from build123d import *

# Parameters (mm, degrees)
SKETCH001_R  = 35
PAD_DEPTH    = 10
FILLET_R     = 3
SKETCH_R     = 33.5
POCKET_DEPTH = 9
FILLET001_R  = 2


with BuildPart() as part:
    # Sketch001 → Pad (new body)
    with BuildSketch(Plane.XY):
        Circle(SKETCH001_R)
    extrude(amount=PAD_DEPTH)

    # Fillet
    fillet_edges = [part.edges().sort_by_distance(p)[0] for p in [
        (-35, 0, 10),
    ]]
    fillet(fillet_edges, radius=FILLET_R)

    # Sketch → Pocket (cut)
    with BuildSketch(Plane.XY):
        Circle(SKETCH_R)
    extrude(amount=POCKET_DEPTH, mode=Mode.SUBTRACT)

    # Fillet001
    fillet001_edges = [part.edges().sort_by_distance(p)[0] for p in [
        (-33.5, 0, 9),
    ]]
    fillet(fillet001_edges, radius=FILLET001_R)


solid = part.part
Geometry check sheet. Reference: the model listing, model coordinates, mm. A direction names the side the tool comes from. Coordinates: 2 decimals unless noted, no trailing zeros. Loops run counter-clockwise (first coordinate to the right, second up) from the corner with the lowest first, then second, coordinate; pieces in that order, holes last. Notation, with made-up numbers: (22.5, 52) - (41.5, 52) arc R19 cw to (41.5, 80) - close; hole circle Ø3 at (78.25, 8). An arc over 180 degrees is marked (long way). Use one line per item in the form item = value. Start each with the question number.
Item 1: Section check A-A, the plane x = 0. Enter the section's corners in (y, z).
Item 2: Gauge pin test, flat ends, axial feed: pin 1 (19 mm diameter, centred on x = 2, y = 3.5, fed in from -Z); pin 2 (1.5 mm diameter, centred on x = 20, z = 5.5, fed in from +Y); pin 3 (1.5 mm diameter, centred on y = 5, z = 2.5, fed in from -X). Record the tip position at first contact, or that the pin passes through.
Item 3: Thickness scan on probe 1 along Y at (x, z) = (0, 2.25); probe 2 along Z at (x, y) = (-5.5, 12); probe 3 along X at (y, z) = (-19, 1). Record the ranges inside material, lowest first.
Item 4: Tool access check on faces 1 (the face through (0, 0, 10)), 2 (the face through (-7.262, -32.703, 3.451)). Record the directions out of +Z, -Z, +X, -X, +Y, -Y that give a thin tool (end or side, any length) a straight path to the whole face; none if there is none.
Item 5: Mould release check, pull along Y, two halves, no side actions. Record for faces 3 (the face through (0, -34, 0)), 4 (the face through (-28, -21, 3)), 5 (the face through (0, 0, 9)): +Y half, -Y half, draft (parallel to the pull), parting line (faces both ways), or undercut.
Computed:
q1.outline = (-35, 0) - (-33.5, 0) - (-33.5, 7) arc R2 cw to (-31.5, 9) - (31.5, 9) arc R2 cw to (33.5, 7) - (33.5, 0) - (35, 0) - (35, 7) arc R3 ccw to (32, 10) - (-32, 10) arc R3 ccw to (-35, 7) - close
q2.pin_1 = 9
q2.pin_2 = 29.23
q2.pin_3 = -34.74
q3.probe_1 = -35 to -33.5, 33.5 to 35
q3.probe_2 = 9 to 10
q3.probe_3 = -29.39 to -27.59, 27.59 to 29.39
q4.face_1 = +Z, +X, -X, +Y, -Y
q4.face_2 = -Z
q5.face_3 = draft
q5.face_4 = parting line
q5.face_5 = undercut
